Work out the finished part from the listing and answer in its coordinate system (mm). Face numbers are marked on the shaded views. A direction names the side the tool comes from. Give positions to 0.01 mm unless a question says otherwise; leave off trailing zeros. Loops run counter-clockwise (first coordinate to the right, second up) from the corner with the lowest first, then second, coordinate; pieces in that order, holes last.
```python
from build123d import *

# Parameters (mm, degrees)
F1_DEPTH = 64.008
F2_W     = 37.431452
F2_H     = 81.391217
F3_DEPTH = 25.4


with BuildPart() as f1:
    # F0 (on Top) → F1 (new body)
    with BuildSketch(Plane.XY):
        Polygon((-43.390859, 22.354396), (-43.390859, -59.036821), (43.390859, -59.036821), (43.390859, 59.036821), align=None)
    extrude(amount=-F1_DEPTH)

    # F2 (on face) → F3 (join)
    with BuildSketch(Plane(origin=(0, 0, -64.008), x_dir=(1, 0, 0), z_dir=(0, 0, -1))):
        with Locations((-62.106585, 18.341212)):
            Rectangle(F2_W, F2_H)
        Polygon((43.390859, -59.036821), (-43.390859, -22.354396), (-80.822311, -22.354396), (43.390859, -76.956891), align=None)
        Polygon((-43.390859, 59.036821), (-43.390859, -22.354396), (43.390859, -59.036821), (43.390859, 59.036821), align=None)
    extrude(amount=F3_DEPTH)


solid = f1.part
```
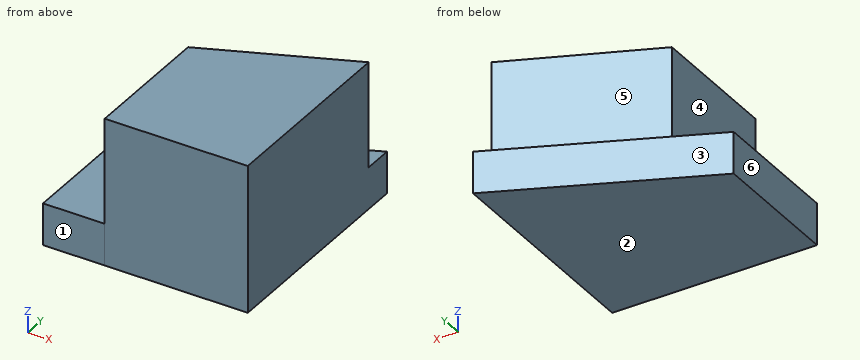
Q1. Section A-A on y = -9 is taken. Give the vertices of the cut face in (x, z).
Q2. Section D-D on x = -62.5 is taken. Give the vertices of the cut face in (y, z).
Q3. Given pin 1 (10 mm diameter, centred on x = -16, z = -46.5, fed in from +Y); pin 2 (12 mm diameter, centred on x = 28.5, z = -31.5, fed in from +Y); pin 3 (1 mm diameter, centred on x = 12.5, y = -25.5, fed in from +Z); pin 4 (2 mm diameter, centred on y = -4.5, z = -21, fed in from -X), each flat-ended and moving along its own axis, determine where each tip first touches the part or whether it passes through.
Q4. Determine the mould class of the marked faces 1, 2 and 3 for opening direction Y: +Y half, -Y half, draft (parallel to the pull), parting line (faces both ways), or undercut.
Q5. Section C-C on z = -38 is taken. Give the vertices of the cut face in (x, y).
Q6. Consider line 1 along Z through (x, y) = (-55.5, -53); line 2 along X through (y, z) = (17, -55); line 3 along Y through (x, z) = (9.5, -80.5). Determine where each line is inside the solid, lowest interval first.
Q7. Section B-B on x = -41 is taken. Give the vertices of the cut face in (y, z) (3 decimals).
Q8. Which of the six approach directions +Z, -Z, +X, -X, +Y, -Y give full straight-line access (tool end or side, diameter ignored) to the marked faces 4, 5 and 6?
Check result:
1. outline: (-80.82, -89.41) - (43.39, -89.41) - (43.39, 0) - (-43.39, 0) - (-43.39, -64.01) - (-80.82, -64.01) - close
2. outline: (-59.04, -89.41) - (30.41, -89.41) - (30.41, -64.01) - (-59.04, -64.01) - close
3. pin 1: stops at y = 36.05
3. pin 2: stops at y = 55.28
3. pin 3: stops at z = 0
3. pin 4: stops at x = -43.39
4. face 1: -Y half
4. face 2: draft
4. face 3: +Y half
5. outline: (-43.39, -59.04) - (43.39, -59.04) - (43.39, 59.04) - (-43.39, 22.35) - close
6. line 1: z = -89.41 to -64.01
6. line 2: x = -43.39 to 43.39
6. line 3: y = -59.04 to 62.06
7. outline: (-59.037, -89.408) - (39.86, -89.408) - (39.86, -64.008) - (23.365, -64.008) - (23.365, 0) - (-59.037, 0) - close
8. face 4: +Z, -X, +Y, -Y
8. face 5: +Z, -X, +Y
8. face 6: +Z, -Z, -X, +Y, -Y
